from build123d import *

# Parameters (mm, degrees)
ESQUISSE1_R             = 20
ESQUISSE1_R_2           = 15
BOSS_EXTRU_1_DEPTH      = 22
ESQUISSE5_R             = 15
BOSS_EXTRU_3_DEPTH      = 2.5
ESQUISSE12_R            = 4.25
ENL_V_MAT_EXTRU_2_DEPTH = 2.5
ESQUISSE13_R            = 1.5
ENL_V_MAT_EXTRU_3_DEPTH = 6


with BuildPart() as part:
    # Esquisse1 → Boss.-Extru.1 (new body)
    with BuildSketch(Plane.XY):
        Circle(ESQUISSE1_R)
        Circle(ESQUISSE1_R_2, mode=Mode.SUBTRACT)
    extrude(amount=BOSS_EXTRU_1_DEPTH)

    # Esquisse5 → Boss.-Extru.3 (add)
    with BuildSketch(Plane(origin=(0, 0, 0), x_dir=(-1, 0, 0), z_dir=(0, 0, -1))):
        Circle(ESQUISSE5_R)
    extrude(amount=-BOSS_EXTRU_3_DEPTH)

    # Esquisse12 → Enlèv. mat.-Extru.2 (cut)
    with BuildSketch(Plane(origin=(0, 0, 0), x_dir=(-1, 0, 0), z_dir=(0, 0, -1))):
        Circle(ESQUISSE12_R)
    extrude(amount=-ENL_V_MAT_EXTRU_2_DEPTH, mode=Mode.SUBTRACT)

    # Esquisse13 → Enlèv. mat.-Extru.3 (cut)
    with BuildSketch(Plane.XY.offset(22)):
        with Locations((16.065617012, 8.273487748)):
            Circle(ESQUISSE13_R)
        with Locations((8.204066222, -16.006302524)):
            Circle(ESQUISSE13_R)
        with Locations((-16.086643669, -8.206225502)):
            Circle(ESQUISSE13_R)
        with Locations((-8.212754961, 16.023254434)):
            Circle(ESQUISSE13_R)
    extrude(amount=-ENL_V_MAT_EXTRU_3_DEPTH, mode=Mode.SUBTRACT)


solid = part.part
Model file for the job. Use its own axes, mm. A direction names the side the tool comes from. Give positions to 0.01 mm unless a question says otherwise; leave off trailing zeros. Order: outer loops, then holes, each group sorted by start corner. A loop starts at its lowest first (then second) coordinate and runs counter-clockwise, first axis right, second up. Notation, with made-up numbers: (-21.75, 73.25) - (6.25, 73.25) arc R32 ccw to (6.25, 100.25) - close; hole circle Ø5 at (82.25, 88.25). An arc over 180 degrees is marked (long way). Write item = value, one per line. Start each with the question number.
1. Which spindle directions (+Z, -Z, +X, -X, +Y, -Y) get a long thin tool onto all of the face, cutting with end or side? Do faces 1 (the flat face through (0, 5, 0)), 2 (the flat face through (-3.12, -3.12, 2.5)). Say none if no direction does.
2. Probe line 1 along Y through (x, z) = (0, 2.05); line 2 along Z through (x, y) = (-5.5, -8); line 3 along X through (y, z) = (-5.5, 2.75). List the from-to ranges inside material, lowest first.
3. Drop flat-ended pins along their axis: P1, Ø1, axis at y = -7.5, z = 7.5, coming from the -X side (3 decimals); P2, Ø2.5, axis at x = 9, y = -16.5, coming from the +Z side; P3, Ø10, axis at y = 10, z = 13, coming from the +X side; P4, Ø2, axis at x = 7, y = 8, coming from the +Z side. Give the stop position or say it passes through.
4. Cut at C-C, the plane y = -9. List the corners of the cut face in (x, z).
5. Cut at D-D, the plane x = 17. List the corners of the cut face in (y, z), and give its area (3 significant figures).
6. Cut at A-A, the plane x = 0. List the corners of the cut face in (y, z).
7. Two-plate mould, pull along X, no slides. Class faces 3 (the cylindrical face through (-2.285, 3.584, 1.232)), 4 (the cylindrical face through (-4.336, -19.524, 10.846)), 5 (the flat face through (-8, -13, 22)): pulls with the +X half, pulls with the -X half, needs draft (parallel to the pull), parting line crosses it, or undercut.
Taken from the geometry:
q1.face_1 = -Z, +X, -X, +Y, -Y
q1.face_2 = +Z
q2.line_1 = -20 to -4.25, 4.25 to 20
q2.line_2 = 0 to 2.5
q2.line_3 = -19.23 to -13.96, 13.96 to 19.23
q3.P1 = -18.735
q3.P2 = 22
q3.P3 = 19.36
q3.P4 = 2.5
q4.outline = (-17.86, 0) - (17.86, 0) - (17.86, 22) - (12, 22) - (12, 2.5) - (-12, 2.5) - (-12, 22) - (-14.81, 22) - (-14.81, 16) - (-17.36, 16) - (-17.36, 22) - (-17.86, 22) - close
q5.outline = (-10.54, 0) - (10.54, 0) - (10.54, 22) - (9.45, 22) - (9.45, 16) - (7.1, 16) - (7.1, 22) - (-10.54, 22) - close
q5.area = 449 mm²
q6.outline = (-20, 0) - (-4.25, 0) - (-4.25, 2.5) - (-15, 2.5) - (-15, 22) - (-20, 22) - close; (4.25, 0) - (20, 0) - (20, 22) - (15, 22) - (15, 2.5) - (4.25, 2.5) - close
q7.face_3 = undercut
q7.face_4 = parting line crosses it
q7.face_5 = needs draft
